```python
from build123d import *

# Parameters (mm, degrees)
CYLINDER006_R          = 10
CYLINDER006_DEPTH      = 100
CYLINDER007_R          = 15
CYLINDER007_DEPTH      = 100
CYLINDER004_R          = 13
CYLINDER004_DEPTH      = 30
CYLINDER005_R          = 20
CYLINDER005_DEPTH      = 40
CUT004_PLACEMENT_ANGLE = 355.865159


with BuildPart() as cylinder006:
    # Cylinder006 → Cylinder006 (new body)
    with BuildSketch(Plane(origin=(50, 0, 150), x_dir=(0, 0, 1), z_dir=(-1, 0, 0))):
        Circle(CYLINDER006_R)
    extrude(amount=CYLINDER006_DEPTH)


with BuildPart() as compound002:
    # Cylinder007 → Cylinder007 (new body)
    with BuildSketch(Plane.ZY.offset(-50)):
        Circle(CYLINDER007_R)
    extrude(amount=CYLINDER007_DEPTH)

    # Compound002: union Cylinder006
    add(cylinder006.part)


with BuildPart() as cone003:
    # Cone001002 → Cone001002 (revolve)
    with BuildSketch(Plane.XZ):
        Polygon((0, 0), (15, 0), (10, 150), (0, 150), align=None)
    revolve(axis=Axis((0, 0, 0), (0, 0, 1)))


with BuildPart() as cylinder004:
    # Cylinder004 → Cylinder004 (new body)
    with BuildSketch(Plane(origin=(15, 0, 150), x_dir=(0, 0, 1), z_dir=(-1, 0, 0))):
        Circle(CYLINDER004_R)
    extrude(amount=CYLINDER004_DEPTH)


with BuildPart() as crank:
    # Cylinder005 → Cylinder005 (new body)
    with BuildSketch(Plane.ZY.offset(-20)):
        Circle(CYLINDER005_R)
    extrude(amount=CYLINDER005_DEPTH)

    # Fusion002: union Cone003, Cylinder004
    add(cone003.part)
    add(cylinder004.part)

    # Cut004: cut Compound002
    add(compound002.part, mode=Mode.SUBTRACT)


with BuildPart() as crank_1:
    # Cut004 placement: moved
    add(crank.part.moved(Location((0, -10.815595, -33.286978))).rotate(Axis((0, -10.815595, -33.286978), (1, 0, 0)), CUT004_PLACEMENT_ANGLE))


solid = crank_1.part
```
Design review of the part built by this model. Coordinates are the model's own, in mm. A direction names the side the tool comes from. Coordinates: 2 decimals unless noted, no trailing zeros.
1) Take a section at A-A, the plane x = -11. State how many separate pieces and enclosed holes the cut face has, and give its area (3 significant figures).
2) Wall thickness on line 1 along Z through (x, y) = (-9.5, 5); line 2 along Z through (x, y) = (-2.5, 0); line 3 along Z through (x, y) = (11, 2): over which ranges is each line inside the solid? List them lowest first.
3) Clearance check with flat-ended pins moving along their axes: pin 1 (4 mm diameter, centred on x = -5, z = 46, fed in from +Y); pin 2 (2 mm diameter, centred on y = 2, z = 46, fed in from -X); pin 3 (21 mm diameter, centred on y = -3, z = 118, fed in from +X). State where each tip first meets the part, or that it passes through.
4) For faces 1 (the flat face through (-15, -7, 124)), 2 (the flat face through (15, -7, 124)), 3 (the flat face through (20, 4.3, -31.5)), list the 3-axis set-ups (+Z, -Z, +X, -X, +Y, -Y) from which the entire face can be reached by the end or side of a thin tool; tool diameter is ignored.
5) Mouldability with a two-part tool opening along Y and no side actions: class faces 4 (the conical face through (6.652, 5.271, 44.531)), 5 (the flat face through (-20, 4.3, -31.5)), 6 (the cylindrical face through (0.28, -15.547, -19.053)) as +Y half, -Y half, draft (parallel to the pull), parting line (faces both ways), or undercut.
Returned:
1. separate pieces: 2
1. enclosed holes: 2
1. area: 1,970 mm2
2. line 1: z = -45.53 to -21.04, 104.32 to 107.66, 124.98 to 128.32
2. line 2: z = -50.11 to -43.68, -22.89 to 106.32, 126.32 to 129.32
2. line 3: z = -48.64 to -41.08, -25.49 to -17.93, 103.48 to 106.52, 126.12 to 129.17
3. pin 1: stops at y = 6.9
3. pin 2: stops at x = -10.74
3. pin 3: stops at x = 15
4. face 1: +Z, -X, +Y, -Y
4. face 2: +Z, +X, +Y, -Y
4. face 3: +Z, -Z, +X, +Y, -Y
5. face 4: parting line
5. face 5: draft
5. face 6: undercut
